Design review of the part built by this model. Coordinates are the model's own, in mm. Coordinates: 2 decimals unless noted, no trailing zeros. Write each loop counter-clockwise with the first axis right and the second up, starting at its lowest first coordinate (ties: lowest second). Pieces come first, ordered by that corner, then holes.
Q1. For pin 1 Ø0.9 at (x, z) = (51.5, 1) entering from -Y; pin 2 Ø1.5 at (y, z) = (54.5, 2) entering from -X; pin 3 Ø5 at (x, y) = (25.5, -7.5) entering from +Z, all flat-tipped, find the tip position at first contact; note any pin that passes through.
Q2. Take a section at C-C, the plane z = 1.6. State how many separate pieces and enclosed holes the cut face has, plus the area to 3 significant figures.
Q3. Take a section at B-B, the plane x = -57. Write out the cut boundary in (y, z), plus the area to 3 significant figures.
Q4. Take a section at A-A, the plane y = -30.5. Write out the cut boundary in (x, z).
Q5. For L1, parallel to Y at x = -60, z = 0.65, list the stretches that pass through material, from the lowest coordinate up.
from build123d import *

# Parameters (mm, degrees)
BOSS_EXTRUDE1_DEPTH = 3
SKETCH2_W           = 17.216666667
SKETCH2_H           = 17.216666667
SKETCH2_W_2         = 17.216666666
SKETCH2_H_2         = 17.216666666
CUT_EXTRUDE1_DEPTH  = 96.011815055


with BuildPart() as part:
    # Sketch1 → Boss-Extrude1 (new body)
    with BuildSketch(Plane.XY):
        Polygon((0, -64.15), (-21.283333333, -64.15), (-21.283333333, -67.15), (-42.866666667, -67.15), (-42.866666667, -64.15), (-64.15, -64.15), (-64.15, -42.866666667), (-67.15, -42.866666667), (-67.15, -21.283333333), (-64.15, -21.283333333), (-64.15, 0), (-64.15, 21.283333333), (-67.15, 21.283333333), (-67.15, 42.866666667), (-64.15, 42.866666667), (-64.15, 64.15), (-42.866666667, 64.15), (-42.866666667, 67.15), (-21.283333333, 67.15), (-21.283333333, 64.15), (0, 64.15), (21.283333333, 64.15), (21.283333333, 67.15), (42.866666667, 67.15), (42.866666667, 64.15), (64.15, 64.15), (64.15, 42.866666667), (67.15, 42.866666667), (67.15, 21.283333333), (64.15, 21.283333333), (64.15, 0), (64.15, -21.283333333), (67.15, -21.283333333), (67.15, -42.866666667), (64.15, -42.866666667), (64.15, -64.15), (42.866666667, -64.15), (42.866666667, -67.15), (21.283333333, -67.15), (21.283333333, -64.15), align=None)
    extrude(amount=BOSS_EXTRUDE1_DEPTH)

    # Sketch2 → Cut-Extrude1 (cut, through all)
    with BuildSketch(Plane.XY.offset(3)):
        with Locations((-50.541666667, 50.541666667)):
            Rectangle(SKETCH2_W, SKETCH2_H)
        with Locations((-30.325, 50.541666667)):
            Rectangle(SKETCH2_W_2, SKETCH2_H)
        with Locations((-10.108333334, 50.541666667)):
            Rectangle(SKETCH2_W, SKETCH2_H)
        with Locations((10.108333334, 50.541666667)):
            Rectangle(SKETCH2_W, SKETCH2_H)
        with Locations((30.325, 50.541666667)):
            Rectangle(SKETCH2_W_2, SKETCH2_H)
        with Locations((50.541666667, 50.541666667)):
            Rectangle(SKETCH2_W, SKETCH2_H)
        with Locations((-30.325, 30.325)):
            Rectangle(SKETCH2_W_2, SKETCH2_H_2)
        with Locations((-10.108333334, 30.325)):
            Rectangle(SKETCH2_W, SKETCH2_H_2)
        with Locations((10.108333334, 30.325)):
            Rectangle(SKETCH2_W, SKETCH2_H_2)
        with Locations((30.325, 30.325)):
            Rectangle(SKETCH2_W_2, SKETCH2_H_2)
        with Locations((50.541666667, 30.325)):
            Rectangle(SKETCH2_W, SKETCH2_H_2)
        with Locations((-30.325, 10.108333334)):
            Rectangle(SKETCH2_W_2, SKETCH2_H)
        with Locations((-10.108333334, 10.108333334)):
            Rectangle(SKETCH2_W, SKETCH2_H)
        with Locations((10.108333334, 10.108333334)):
            Rectangle(SKETCH2_W, SKETCH2_H)
        with Locations((30.325, 10.108333334)):
            Rectangle(SKETCH2_W_2, SKETCH2_H)
        with Locations((50.541666667, 10.108333334)):
            Rectangle(SKETCH2_W, SKETCH2_H)
        with Locations((-30.325, -10.108333334)):
            Rectangle(SKETCH2_W_2, SKETCH2_H)
        with Locations((-10.108333334, -10.108333334)):
            Rectangle(SKETCH2_W, SKETCH2_H)
        with Locations((10.108333334, -10.108333334)):
            Rectangle(SKETCH2_W, SKETCH2_H)
        with Locations((30.325, -10.108333334)):
            Rectangle(SKETCH2_W_2, SKETCH2_H)
        with Locations((50.541666667, -10.108333334)):
            Rectangle(SKETCH2_W, SKETCH2_H)
        with Locations((-30.325, -30.325)):
            Rectangle(SKETCH2_W_2, SKETCH2_H_2)
        with Locations((-10.108333334, -30.325)):
            Rectangle(SKETCH2_W, SKETCH2_H_2)
        with Locations((10.108333334, -30.325)):
            Rectangle(SKETCH2_W, SKETCH2_H_2)
        with Locations((30.325, -30.325)):
            Rectangle(SKETCH2_W_2, SKETCH2_H_2)
        with Locations((50.541666667, -30.325)):
            Rectangle(SKETCH2_W, SKETCH2_H_2)
        with Locations((-30.325, -50.541666667)):
            Rectangle(SKETCH2_W_2, SKETCH2_H)
        with Locations((-10.108333334, -50.541666667)):
            Rectangle(SKETCH2_W, SKETCH2_H)
        with Locations((10.108333334, -50.541666667)):
            Rectangle(SKETCH2_W, SKETCH2_H)
        with Locations((30.325, -50.541666667)):
            Rectangle(SKETCH2_W_2, SKETCH2_H)
        with Locations((50.541666667, -50.541666667)):
            Rectangle(SKETCH2_W, SKETCH2_H)
        with Locations((-50.541666667, 30.325)):
            Rectangle(SKETCH2_W, SKETCH2_H_2)
        with Locations((-50.541666667, 10.108333334)):
            Rectangle(SKETCH2_W, SKETCH2_H)
        with Locations((-50.541666667, -10.108333334)):
            Rectangle(SKETCH2_W, SKETCH2_H)
        with Locations((-50.541666667, -30.325)):
            Rectangle(SKETCH2_W, SKETCH2_H_2)
        with Locations((-50.541666667, -50.541666667)):
            Rectangle(SKETCH2_W, SKETCH2_H)
    extrude(amount=-CUT_EXTRUDE1_DEPTH, mode=Mode.SUBTRACT)


solid = part.part
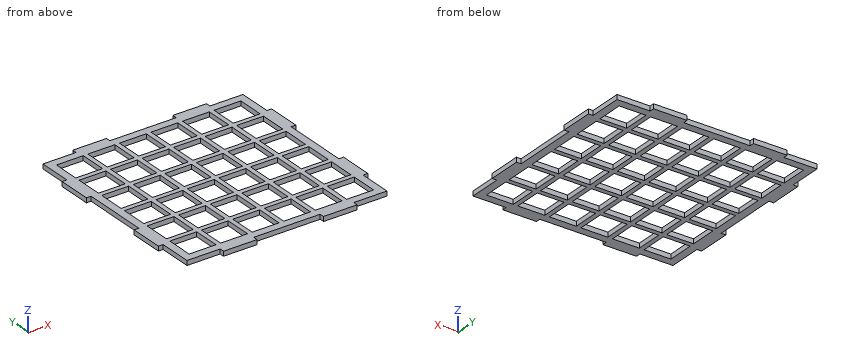
Responses:
1. pin 1: stops at y = -64.15
1. pin 2: stops at x = -64.15
1. pin 3: passes through
2. separate pieces: 1
2. enclosed holes: 36
2. area: 6,310 mm2
3. outline: (-64.15, 0) - (-59.15, 0) - (-59.15, 3) - (-64.15, 3) - close; (-41.93, 0) - (-38.93, 0) - (-38.93, 3) - (-41.93, 3) - close; (-21.72, 0) - (-18.72, 0) - (-18.72, 3) - (-21.72, 3) - close; (-1.5, 0) - (1.5, 0) - (1.5, 3) - (-1.5, 3) - close; (18.72, 0) - (21.72, 0) - (21.72, 3) - (18.72, 3) - close; (38.93, 0) - (41.93, 0) - (41.93, 3) - (38.93, 3) - close; (59.15, 0) - (64.15, 0) - (64.15, 3) - (59.15, 3) - close
3. area: 75.0 mm2
4. outline: (-67.15, 0) - (-59.15, 0) - (-59.15, 3) - (-67.15, 3) - close; (-41.93, 0) - (-38.93, 0) - (-38.93, 3) - (-41.93, 3) - close; (-21.72, 0) - (-18.72, 0) - (-18.72, 3) - (-21.72, 3) - close; (-1.5, 0) - (1.5, 0) - (1.5, 3) - (-1.5, 3) - close; (18.72, 0) - (21.72, 0) - (21.72, 3) - (18.72, 3) - close; (38.93, 0) - (41.93, 0) - (41.93, 3) - (38.93, 3) - close; (59.15, 0) - (67.15, 0) - (67.15, 3) - (59.15, 3) - close
5. L1: y = -64.15 to 64.15
